```python
from build123d import *

# Parameters (mm, degrees)
F0_W      = 54
F0_H      = 89
F1_DEPTH  = 1.7
F2_W      = 3
F2_H      = 83
F3_DEPTH  = 4
F4_W      = 6
F4_H      = 6
F5_DEPTH  = 3.5
F7_R      = 2.5
F6_R      = 2.5
F8_DEPTH  = 6
F9_W      = 2
F9_H      = 3
F10_DEPTH = 2
F11_W     = 9
F11_H     = 7
F11_H_2   = 2
F12_DEPTH = 4
F13_W     = 3
F13_H     = 3
F13_W_2   = 2
F14_DEPTH = 2


with BuildPart() as f1:
    # F0 (on Top) → F1 (new body)
    with BuildSketch(Plane.XY):
        with Locations((27, 44.5)):
            Rectangle(F0_W, F0_H)
    extrude(amount=F1_DEPTH)

    # F2 (on face) → F3 (join)
    with BuildSketch(Plane.XY.offset(1.7)):
        with Locations((7.5, 44.5)):
            Rectangle(F2_W, F2_H)
        with Locations((46.5, 44.5)):
            Rectangle(F2_W, F2_H)
    extrude(amount=F3_DEPTH)

    # F4 (on face) → F5 (join)
    with BuildSketch(Plane.XY.offset(1.7)):
        with Locations((18.2, 20)):
            Rectangle(F4_W, F4_H)
        with Locations((35.8, 20)):
            Rectangle(F4_W, F4_H)
    extrude(amount=F5_DEPTH)

    # F7 (on face) + F6 (on face) → F8 (join)
    with BuildSketch(Plane.XY.offset(5.2)):
        with Locations((35.8, 20)):
            Circle(F7_R)
    with BuildSketch(Plane.XY.offset(5.2)):
        with Locations((18.2, 20)):
            Circle(F6_R)
    extrude(amount=F8_DEPTH)

    # F9 (on face) → F10 (join)
    with BuildSketch(Plane.XY.offset(1.7)):
        with Locations((42.5, 11)):
            Rectangle(F9_W, F9_H)
        with Locations((11.5, 11)):
            Rectangle(F9_W, F9_H)
    extrude(amount=F10_DEPTH)

    # F11 (on face) → F12 (join)
    with BuildSketch(Plane.XY.offset(1.7)):
        with Locations((27, 85.5)):
            Rectangle(F11_W, F11_H)
        with Locations((27, 90)):
            Rectangle(F11_W, F11_H_2)
    extrude(amount=F12_DEPTH)

    # F13 (on face) → F14 (join)
    with BuildSketch(Plane.XY.offset(1.7)):
        with Locations((14.5, 83.3)):
            Rectangle(F13_W, F13_H)
        with Locations((38.5, 86.5)):
            Rectangle(F13_W_2, F13_H)
    extrude(amount=F14_DEPTH)


solid = f1.part
```
Input: part model. Units: mm. Frame: model coordinates. A direction names the side the tool comes from. Coordinates: 2 decimals unless noted, no trailing zeros. Loops run counter-clockwise (first coordinate to the right, second up) from the corner with the lowest first, then second, coordinate; pieces in that order, holes last. Notation, with made-up numbers: M 4.5,74.5 L 32.5,74.5 A27 cw 32.5,107.5 Z; hole C 56.25,3.25 d2. An arc over 180 degrees is marked long. Use a Markdown table: item, result. Add a question column.
1) Pin query (flat end, axial travel): P1, Ø0.9, axis at x = 7, z = 3, coming from the +Y side; P2, Ø1.5, axis at y = 23, z = 2.5, coming from the -X side; P3, Ø12, axis at x = 47.5, y = 28.5, coming from the -Z side; P4, Ø1, axis at y = 19, z = 3.5, coming from the +X side. Return the tip coordinate at first contact, or that it passes through.
2) Section A-A, the plane y = 20. Return the cut outline in (x, z), plus the area to 3 significant figures.
3) Section D-D, the plane y = 31. Return the cut outline in (x, z).
4) Section B-B, the plane x = 35.8. Return the cut outline in (y, z).
5) Line query: L1, parallel to X at y = 45.5, z = 3.75; L2, parallel to Z at x = 24.5, y = 34; L3, parallel to Y at x = 24.5, z = 3. Output: solid intervals per line, ascending. Write a range as from..to.
6) Set-up query: faces 4 (the flat face through (16, 83, 3)), 5 (the flat face through (21.2, 20, 3)), 6 (the flat face through (27, 90, 1.7)). Return all of +Z, -Z, +X, -X, +Y, -Y with unobstructed straight access to the full face (end or side cutting, diameter ignored); none if empty.
7) Draft query along X for faces 1 (the flat face through (15.2, 20, 3)), 2 (the flat face through (0, 44, 1)), 3 (the flat face through (7, 3, 4)). Return one class per face: +X half, -X half, draft (parallel to the pull), parting line (faces both ways), or undercut.
8) Section C-C, the plane z = 7. Return the cut outline in (x, y).
Answer below:
| question | item | result |
|---|---|---|
| 1 | P1 | y = 86 |
| 1 | P2 | x = 6 |
| 1 | P3 | z = 0 |
| 1 | P4 | x = 48 |
| 2 | outline | M 0,0 L 54,0 L 54,1.7 L 48,1.7 L 48,5.7 L 45,5.7 L 45,1.7 L 38.8,1.7 L 38.8,5.2 L 38.3,5.2 L 38.3,11.2 L 33.3,11.2 L 33.3,5.2 L 32.8,5.2 L 32.8,1.7 L 21.2,1.7 L 21.2,5.2 L 20.7,5.2 L 20.7,11.2 L 15.7,11.2 L 15.7,5.2 L 15.2,5.2 L 15.2,1.7 L 9,1.7 L 9,5.7 L 6,5.7 L 6,1.7 L 0,1.7 Z |
| 2 | area | 218 mm2 |
| 3 | outline | M 0,0 L 54,0 L 54,1.7 L 48,1.7 L 48,5.7 L 45,5.7 L 45,1.7 L 9,1.7 L 9,5.7 L 6,5.7 L 6,1.7 L 0,1.7 Z |
| 4 | outline | M 0,0 L 89,0 L 89,1.7 L 23,1.7 L 23,5.2 L 22.5,5.2 L 22.5,11.2 L 17.5,11.2 L 17.5,5.2 L 17,5.2 L 17,1.7 L 0,1.7 Z |
| 5 | L1 | 6..9, 45..48 |
| 5 | L2 | 0..1.7 |
| 5 | L3 | 82..91 |
| 6 | face 4 | +Z, +Y |
| 6 | face 5 | +Z, +Y, -Y |
| 6 | face 6 | -Z, +X, -X, +Y |
| 7 | face 1 | undercut |
| 7 | face 2 | -X half |
| 7 | face 3 | draft |
| 8 | outline | C 18.2,20 d5; C 35.8,20 d5 |
